Geometry: see drawing. Coordinates: mm, zero at the bounding-box minimum. A direction names the side the tool comes from. Coordinates: 2 decimals unless noted, no trailing zeros. Loops run counter-clockwise (first coordinate to the right, second up) from the corner with the lowest first, then second, coordinate; pieces in that order, holes last. Notation, with made-up numbers: (1.25, 85) -> (12.25, 85) arc R28 ccw to (12.25, 106) -> close; hole circle Ø7 at (-11, 34.25). An arc over 180 degrees is marked (long way). Put each result on its own line as item: value. Start each with the question number.
1) Cut plane D-D (x = 32.5). Return the cut outline in (y, z), plus the area to 3 significant figures.
2) Contact query for flat-ended pins moving along their axis: P1, Ø10, axis at x = 31, y = 10.5, coming from the +Z side; P2, Ø4, axis at x = 22.5, y = 22.5, coming from the -Z side; P3, Ø5.5, axis at y = 30, z = 30, coming from the +X side; P4, Ø4.5, axis at y = 29.5, z = 9.5, coming from the +X side. Output: stop coordinate, or through.
3) Material intervals for L1, parallel to X at y = 7.25, z = 17.5 (3 decimals); L2, parallel to Z at x = 5, y = 30 (3 decimals); L3, parallel to Z at x = 5, y = 26.5 (3 decimals), sorted ascending.
4) Set-up query: the marked faces 5, 6 and 7. Return all of +Z, -Z, +X, -X, +Y, -Y with unobstructed straight access to the full face (end or side cutting, diameter ignored); none if empty.
5) Cut plane A-A (x = 5). Return the cut outline in (y, z) (3 decimals).
6) Cut plane C-C (z = 17.5). Return the cut outline in (x, y) (3 decimals), plus the area to 3 significant figures.
7) Pull-direction query (X, two-part tool) for the marked faces 1, 2, 3 and 4; classes: pulls with the +X half, pulls with the -X half, needs draft (parallel to the pull), parting line crosses it, or undercut.
8) Cut plane B-B (y = 25.5). Return the cut outline in (x, z) (3 decimals), plus the area to 3 significant figures.
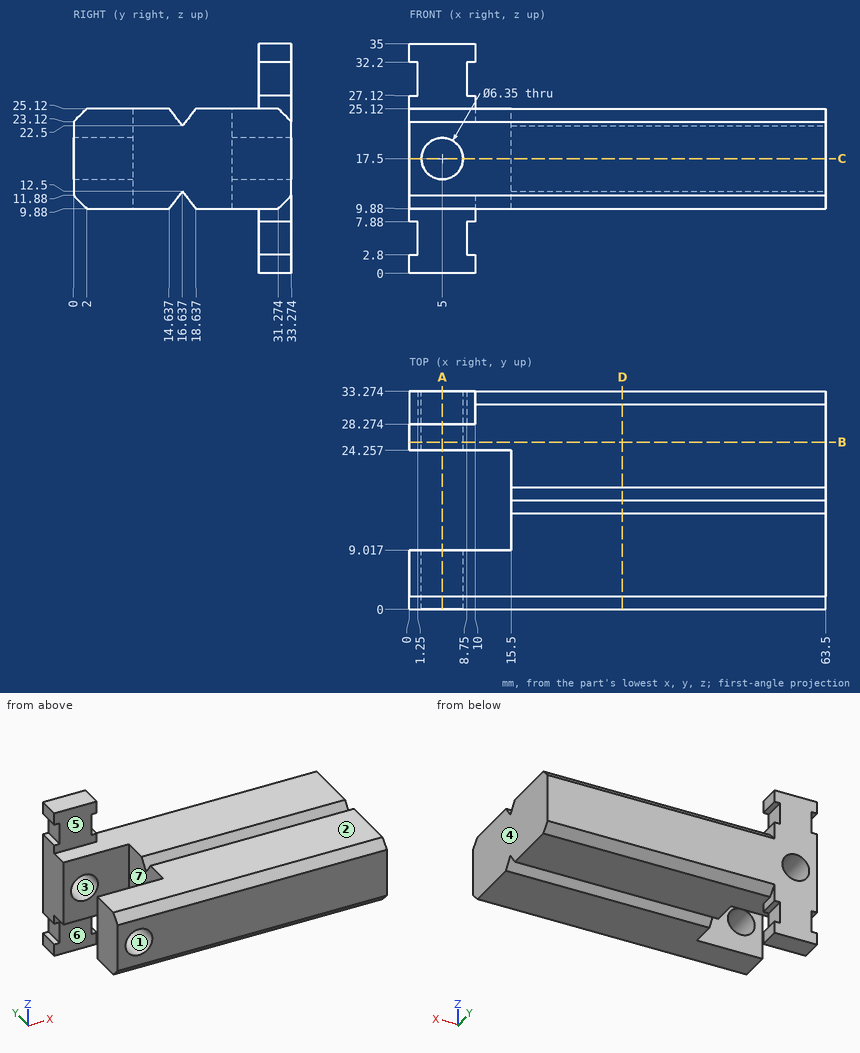
Results found:
1. outline: (0, 11.88) -> (2, 9.88) -> (14.64, 9.88) -> (16.64, 12.5) -> (18.64, 9.88) -> (31.27, 9.88) -> (33.27, 11.88) -> (33.27, 23.12) -> (31.27, 25.12) -> (18.64, 25.12) -> (16.64, 22.5) -> (14.64, 25.12) -> (2, 25.12) -> (0, 23.12) -> close
1. area: 489 mm2
2. P1: stops at z = 25.12
2. P2: stops at z = 9.88
2. P3: stops at x = 10
2. P4: stops at x = 63.5
3. L1: x = 0 to 1.825, 8.175 to 63.5
3. L2: z = 0 to 14.325, 20.675 to 35
3. L3: z = 9.88 to 14.325, 20.675 to 25.12
4. face 5: +Z, +X, -X, -Y
4. face 6: -Z, +X, -X, -Y
4. face 7: +Z, -Z, -X
5. outline: (0, 11.88) -> (2, 9.88) -> (9.017, 9.88) -> (9.017, 14.325) -> (0, 14.325) -> close; (0, 20.675) -> (9.017, 20.675) -> (9.017, 25.12) -> (2, 25.12) -> (0, 23.12) -> close; (24.257, 9.88) -> (28.274, 9.88) -> (28.274, 0) -> (33.274, 0) -> (33.274, 14.325) -> (24.257, 14.325) -> close; (24.257, 20.675) -> (33.274, 20.675) -> (33.274, 35) -> (28.274, 35) -> (28.274, 25.12) -> (24.257, 25.12) -> close
6. outline: (0, 0) -> (1.825, 0) -> (1.825, 9.017) -> (0, 9.017) -> close; (0, 24.257) -> (1.825, 24.257) -> (1.825, 33.274) -> (0, 33.274) -> close; (8.175, 0) -> (63.5, 0) -> (63.5, 33.274) -> (8.175, 33.274) -> (8.175, 24.257) -> (15.5, 24.257) -> (15.5, 9.017) -> (8.175, 9.017) -> close
6. area: 1,760 mm2
7. face 1: undercut
7. face 2: needs draft
7. face 3: undercut
7. face 4: pulls with the +X half
8. outline: (0, 9.88) -> (63.5, 9.88) -> (63.5, 25.12) -> (0, 25.12) -> close; hole circle Ø6.35 at (5, 17.5)
8. area: 936 mm2
